Part model, mm, in its own coordinate system. Face numbers are marked on the shaded views. A direction names the side the tool comes from. Give positions to 0.01 mm unless a question says otherwise; leave off trailing zeros. Write each loop counter-clockwise with the first axis right and the second up, starting at its lowest first coordinate (ties: lowest second). Pieces come first, ordered by that corner, then holes. Notation, with made-up numbers: (-1.5, -1) - (24.5, -1) arc R17 ccw to (24.5, 13) - close; hole circle Ø10 at (-26.75, 82). An arc over 180 degrees is marked (long way). Answer as a JSON object with one key per item and string values. Group by question number.
```python
from build123d import *

# Parameters (mm, degrees)
F0_W      = 15
F0_H      = 33
F1_DEPTH  = 3
F3_W      = 2.4
F3_H      = 1.2
F4_DEPTH  = 1.2
F7_DEPTH  = 1.2
F9_ANGLE  = 180
F11_ANGLE = 180
F15_ANGLE = 180
F16_ANGLE = 180
F18_ANGLE = 180
F19_ANGLE = 115
F20_ANGLE = 180
F2_W      = 15
F2_H      = 33
F2_W_2    = 13
F2_H_2    = 31
F21_DEPTH = 1


with BuildPart() as f1:
    # F0 (on Top) → F1 (new body)
    with BuildSketch(Plane.XY):
        with Locations((7.5, 16.5)):
            Rectangle(F0_W, F0_H)
        with BuildLine():
            ThreePointArc((15, 33), (7.5, 40.5), (0, 33))
            Line((0, 33), (15, 33))
        make_face()
        with BuildLine():
            Line((11.4686269666, 35), (3.5313730334, 35))
            ThreePointArc((3.5313730334, 35), (2.9126545999, 35.3726049787), (2.9526149341, 36.09375))
            ThreePointArc((2.9526149341, 36.09375), (7.5, 38.5), (12.0473850659, 36.09375))
            ThreePointArc((12.0473850659, 36.09375), (12.0873454001, 35.3726049787), (11.4686269666, 35))
        make_face(mode=Mode.SUBTRACT)
    extrude(amount=F1_DEPTH)

    # F3 (on face) → F4 (join)
    with BuildSketch(Plane.XY.offset(3)):
        with Locations((4.4729229599, 8.7)):
            Rectangle(F3_W, F3_H)
        Polygon((2.9330339742, 7.8), (1.7330344026, 7.801014062), (1.7310062787, 5.4010149189), (2.9310058502, 5.4000008569), align=None)
        Polygon((7.6412468567, 6.8621327115), (6.7072128218, 7.2193167279), (5.9928447889, 5.3512486581), (6.9268788238, 4.9940646416), align=None)
        Polygon((6.1065359398, 3.762840498), (5.5605625677, 4.6), (3.8578521609, 3.4895371309), (4.4313145482, 2.6703052404), align=None)
        Polygon((9.4921899433, 7.8298745016), (8.5952991901, 7.0326374121), (10.189773369, 5.2388559057), (11.0866641222, 6.0360929952), align=None)
        Polygon((9.0970460407, 2.6836514835), (10.8872594075, 3.9623758874), (10.189773369, 4.9388559057), (8.3995600022, 3.6601315018), align=None)
    extrude(amount=F4_DEPTH)

    # F6 (on face) → F7 (join)
    with BuildSketch(Plane.XY.offset(3)):
        Polygon((8.6297593251, 23.3283319113), (10.5786629425, 18.5073595312), (11.9693280521, 19.069543267), (10.0204244347, 23.8905156471), align=None)
        Polygon((9.485872163, 10.4485981269), (11.9552081585, 15.0248826178), (10.6351260938, 15.737191078), (8.1657900983, 11.1609065871), align=None)
    extrude(amount=F7_DEPTH)

    # F8 (on face) → F9 (revolve)
    with BuildSketch(Plane.XY.offset(3)):
        with BuildLine():
            Line((11.9, 18.6), (11.9, 15.6))
            ThreePointArc((11.9, 15.6), (13.4, 17.1), (11.9, 18.6))
        make_face()
    revolve(axis=Axis((11.9, 17.1, 3), (0, -1, 0)), revolution_arc=F9_ANGLE)

    # F10 (on face) → F11 (revolve)
    with BuildSketch(Plane.XY.offset(3)):
        with BuildLine():
            Line((8.15, 28.55), (8.15, 23.85))
            ThreePointArc((8.15, 23.85), (10.5, 26.2), (8.15, 28.55))
        make_face()
    revolve(axis=Axis((8.15, 26.2, 3), (0, -1, 0)), revolution_arc=F11_ANGLE)

    # F14 (on face) → F15 (revolve)
    with BuildSketch(Plane.XY.offset(3)):
        with BuildLine():
            Line((2.4674874008, 9.2003644818), (2.4674874008, 8.0004137249))
            ThreePointArc((2.4674874008, 8.0004137249), (3.0729229599, 8.6003891034), (2.4674874008, 9.2003644818))
        make_face()
    revolve(axis=Axis((2.4674874008, 8.6003891034, 3), (0, -1, 0)), revolution_arc=F15_ANGLE)

    # F13 (on face) → F16 (revolve)
    with BuildSketch(Plane.XY.offset(3)):
        with BuildLine():
            Line((6.3335492538, 5.0726566499), (6.3335492538, 4.0726566499))
            ThreePointArc((6.3335492538, 4.0726566499), (6.8335492538, 4.5726566499), (6.3335492538, 5.0726566499))
        make_face()
    revolve(axis=Axis((6.3335492538, 4.5726566499, 3), (0, -1, 0)), revolution_arc=F16_ANGLE)

    # F17 (on face) → F18 (revolve)
    with BuildSketch(Plane.XY.offset(3)):
        with BuildLine():
            Line((11.2385163883, 5.5374744504), (11.2385163883, 4.3374744504))
            ThreePointArc((11.2385163883, 4.3374744504), (11.8385163883, 4.9374744504), (11.2385163883, 5.5374744504))
        make_face()
    revolve(axis=Axis((11.2385163883, 4.9374744504, 3), (0, -1, 0)), revolution_arc=F18_ANGLE)

    # F12 (on face) → F19 (revolve)
    with BuildSketch(Plane.XY.offset(3)):
        with BuildLine():
            Line((4.9804255393, 24.7154806374), (11.3195744607, 27.6845193626))
            ThreePointArc((11.3195744607, 27.6845193626), (6.6654806374, 29.3695744607), (4.9804255393, 24.7154806374))
        make_face()
    revolve(axis=Axis((8.15, 26.2, 3), (0.9055927031, 0.4241483893, 0)), revolution_arc=F19_ANGLE)

    # F5 (on face) → F20 (revolve)
    with BuildSketch(Plane.XY.offset(3)):
        with BuildLine():
            Line((7.75, 10.75), (7.75, 7.25))
            ThreePointArc((7.75, 7.25), (9.5, 9), (7.75, 10.75))
        make_face()
    revolve(axis=Axis((7.75, 9, 3), (0, -1, 0)), revolution_arc=F20_ANGLE)

    # F2 (on face) → F21 (join)
    with BuildSketch(Plane.XY.offset(3)):
        with Locations((7.5, 16.5)):
            Rectangle(F2_W, F2_H)
        with Locations((7.5, 16.5)):
            Rectangle(F2_W_2, F2_H_2, mode=Mode.SUBTRACT)
    extrude(amount=F21_DEPTH)


solid = f1.part
```
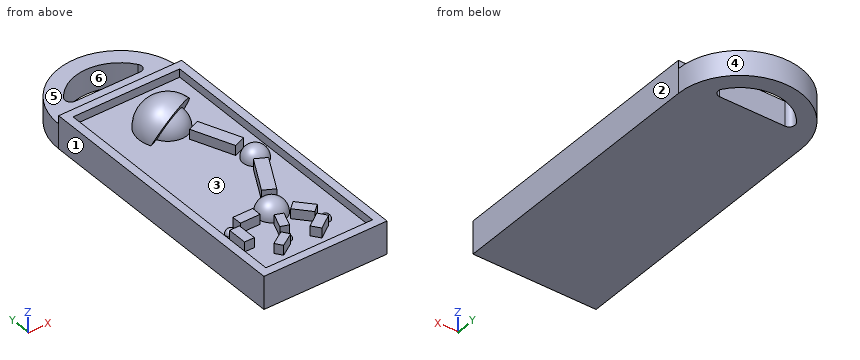
1) Drop flat-ended pins along their axis: P1, Ø0.6, axis at x = 4, z = 3.5, coming from the +Y side; P2, Ø6, axis at x = 6.5, y = 31.5, coming from the +Z side; P3, Ø1, axis at x = 2.5, y = 6.5, coming from the +Z side; P4, Ø3, axis at y = 16, z = 4.5, coming from the +X side. Give the stop position or say it passes through.
2) Mould opens along X. For the marked faces 1, 2 and 3 say: pulls with the +X half, pulls with the -X half, needs draft (parallel to the pull), parting line crosses it, or undercut.
3) Which spindle directions (+Z, -Z, +X, -X, +Y, -Y) get a long thin tool onto all of the face, cutting with end or side? Do the marked faces 4, 5 and 6. Say none if no direction does.
4) Band-saw the part on A-A (z = 2.25). List the corners of the cut face in (x, y), plus the area to 3 significant figures.
5) Band-saw the part on B-B (y = 22.5). List the corners of the cut face in (x, z), plus the area to 3 significant figures.
6) Band-saw the part on C-C (y = 6.5). List the corners of the cut face in (x, z), plus the area to 3 significant figures.
7) Probe line 1 (Z direction, x = 8, y = 5); line 2 (Z direction, x = 8.75, y = 32.5); line 3 (Y direction, x = 10.5, z = 1). List the from-to ranges inside material, lowest first.
8) Band-saw the part on D-D (y = 14.5). List the corners of the cut face in (x, z).
Verdict:
{
 "1": {"P1": "y = 33", "P2": "z = 5.4", "P3": "z = 4.2", "P4": "x = 15"},
 "2": {"face 1": "pulls with the -X half", "face 2": "pulls with the +X half", "face 3": "undercut"},
 "3": {"face 4": "+Z, -Z, +Y", "face 5": "+Z, +X, -X, +Y", "face 6": "+Z, -Z"},
 "4": {"outline": "(0, 0) - (15, 0) - (15, 33) arc R7.5 ccw to (0, 33) - close; hole (2.95, 36.09) arc R0.7 ccw to (3.53, 35) - (11.47, 35) arc R0.7 ccw to (12.05, 36.09) arc R5.5 ccw to start", "area": "558 mm2"},
 "5": {"outline": "(0, 0) - (15, 0) - (15, 4) - (14, 4) - (14, 3) - (10.58, 3) - (10.58, 4.2) - (8.96, 4.2) - (8.96, 3) - (1, 3) - (1, 4) - (0, 4) - close", "area": "48.9 mm2"},
 "6": {"outline": "(0, 0) - (15, 0) - (15, 4) - (14, 4) - (14, 3) - (10.67, 3) - (10.67, 4.2) - (9.07, 4.2) - (9.07, 3) - (7.5, 3) - (7.5, 4.2) - (6.43, 4.2) - (6.43, 3) - (2.93, 3) - (2.93, 4.2) - (1.73, 4.2) - (1.73, 3) - (1, 3) - (1, 4) - (0, 4) - close", "area": "51.7 mm2"},
 "7": {"line 1": "0 to 3", "line 2": "0 to 4", "line 3": "0 to 35, 37.61 to 39.87"},
 "8": {"outline": "(0, 0) - (15, 0) - (15, 4) - (14, 4) - (14, 3) - (11.67, 3) - (11.67, 4.2) - (9.97, 4.2) - (9.97, 3) - (1, 3) - (1, 4) - (0, 4) - close"}
}
